Verification items for the finished model (mm, model axes). Round coordinates to 2 decimals unless told otherwise and drop trailing zeros. Write each loop counter-clockwise with the first axis right and the second up, starting at its lowest first coordinate (ties: lowest second). Pieces come first, ordered by that corner, then holes. Notation, with made-up numbers: M 29,42.25 L 33,42.25 A24 cw 33,58.25 Z; hole C 10,-32 d3. An arc over 180 degrees is marked long. One line per item, written item: value. Start each with the question number.
Item 1: Section check C-C, the plane z = 10.5. Record the cut outline in (x, y).
Item 2: Section check A-A, the plane z = 2.5. Record the cut outline in (x, y) (1 decimal).
Item 3: Section check D-D, the plane x = 2. Record the cut outline in (y, z).
Item 4: Section check B-B, the plane y = -16. Record the cut outline in (x, z).
Item 5: Thickness scan on probe 1 along Y at (x, z) = (18.5, 2.75); probe 2 along Z at (x, y) = (5.5, -48.5); probe 3 along X at (y, z) = (1, 1.75). Record the ranges inside material, lowest first. Write a range as from..to.
Item 6: Gauge pin test, flat ends, axial feed: pin 1 (8 mm diameter, centred on y = -20.5, z = 10, fed in from +X); pin 2 (6 mm diameter, centred on x = 42, z = 4, fed in from +Y); pin 3 (2 mm diameter, centred on y = -23, z = 11.5, fed in from +X); pin 4 (5 mm diameter, centred on y = -9, z = 3.5, fed in from -X). Record the tip position at first contact, or that the pin passes through.
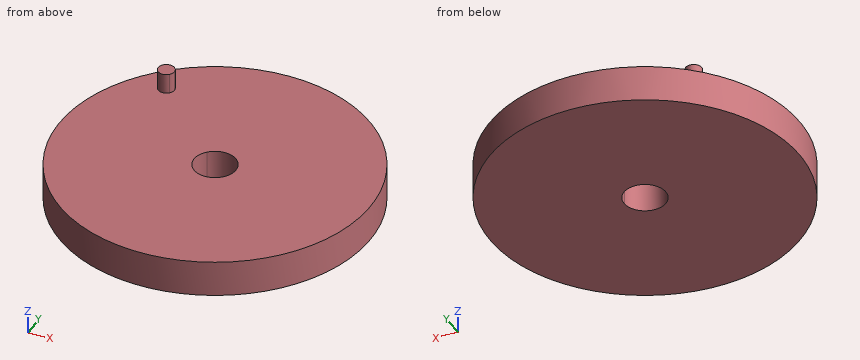
from build123d import *

# Parameters (mm, degrees)
F0_R     = 38.99223
F1_DEPTH = 9.144
F2_DEPTH = 14.224


with BuildPart() as f1:
    # F0 (on Top) → F1 (new body)
    with BuildSketch(Plane.XY):
        with Locations((18.216823, -16.966983)):
            Circle(F0_R)
        with BuildLine():
            ThreePointArc((-3.451107, 5.106916), (-3.592274, 4.362754), (-3.996163, 3.721989))
            ThreePointArc((-3.996163, 3.721989), (-7.373939, 5.851077), (-3.451107, 5.106916))
        make_face(mode=Mode.SUBTRACT)
        with BuildLine():
            ThreePointArc((14.365916, -13.380283), (20.144063, -12.07008), (23.479323, -16.966983))
            ThreePointArc((23.479323, -16.966983), (16.289584, -21.863885), (14.365916, -13.380283))
        make_face(mode=Mode.SUBTRACT)
        with BuildLine():
            ThreePointArc((-3.451107, 5.106916), (-7.373939, 5.851077), (-3.996163, 3.721989))
            ThreePointArc((-3.996163, 3.721989), (-3.592274, 4.362754), (-3.451107, 5.106916))
        make_face()
    extrude(amount=F1_DEPTH)

    # F0 (on Top) → F2 (join)
    with BuildSketch(Plane.XY):
        with BuildLine():
            ThreePointArc((-3.451107, 5.106916), (-7.373939, 5.851077), (-3.996163, 3.721989))
            ThreePointArc((-3.996163, 3.721989), (-3.592274, 4.362754), (-3.451107, 5.106916))
        make_face()
    extrude(amount=F2_DEPTH)


solid = f1.part
Response values:
1. outline: M -4,3.72 A2.03 ccw -3.45,5.11 A2.03 ccw long Z
2. outline: C 18.2,-17 d78; hole C 18.2,-17 d10.5
3. outline: M -52.43,0 L 18.49,0 L 18.49,9.14 L -52.43,9.14 Z
4. outline: M -20.76,0 L 13.04,0 L 13.04,9.14 L -20.76,9.14 Z; M 23.39,0 L 57.2,0 L 57.2,9.14 L 23.39,9.14 Z
5. probe 1: y = -55.96..-22.22, -11.71..22.02
5. probe 2: z = 0..9.14
5. probe 3: x = -16.39..52.82
6. pin 1: stops at x = 57.21
6. pin 2: stops at y = 16.02
6. pin 3: passes through
6. pin 4: stops at x = -20.39
